Could you check a few things on this model? Use its own coordinates, in mm. Face numbers are marked on the shaded views. Coordinates: 2 decimals unless noted, no trailing zeros. Loops run counter-clockwise (first coordinate to the right, second up) from the corner with the lowest first, then second, coordinate; pieces in that order, holes last. Notation, with made-up numbers: (19.5, -4) -> (38.5, -4) arc R23 cw to (38.5, 8) -> close; hole circle Ø3 at (-4.75, 3). An arc over 180 degrees is marked (long way). One line per question, with ' | ' between items.
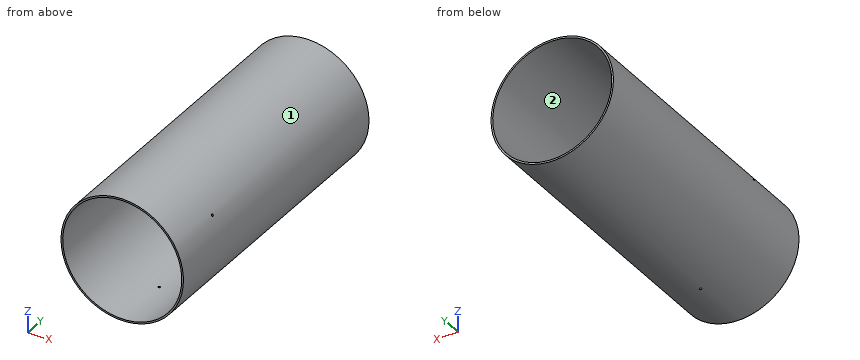
from build123d import *

# Parameters (mm, degrees)
SKETCH1_R               = 78.359
SKETCH1_R_2             = 76.2
BOSS_EXTRUDE1_DEPTH     = 381
CUT_EXTRUDE1_REACH      = 398.789
CUT_EXTRUDE1_END_RADIUS = 78.359
SKETCH2_R               = 1.41224
CIRPATTERN1_COUNT       = 3


with BuildPart() as part:
    # Sketch1 → Boss-Extrude1 (new body)
    with BuildSketch(Plane(origin=(0, 0, 0), x_dir=(1, 0, 0), z_dir=(0, 1, 0))):
        with Locations(Location((0, 0, 0), (0, 0, 270))):
            Circle(SKETCH1_R)
        with Locations(Location((0, 0, 0), (0, 0, 270))):
            Circle(SKETCH1_R_2, mode=Mode.SUBTRACT)
    extrude(amount=BOSS_EXTRUDE1_DEPTH)

    # Cut-Extrude1: up to this cylinder (the profile starts inside it)
    cut_extrude1_end = Plane(origin=(0, 76.2, 0), z_dir=(0, -1, 0)) * Cylinder(CUT_EXTRUDE1_END_RADIUS, 955.296, mode=Mode.PRIVATE)
    # Sketch2 → Cut-Extrude1 (cut, up to the surface)
    with BuildSketch(Plane.XY, mode=Mode.PRIVATE) as cut_extrude1_sk1:
        with Locations((0, 76.2)):
            Circle(SKETCH2_R)
    cut_extrude1_tool1 = extrude(cut_extrude1_sk1.sketch, amount=-CUT_EXTRUDE1_REACH, mode=Mode.PRIVATE) & cut_extrude1_end
    cut_extrude1 = cut_extrude1_tool1.solids().sort_by_distance((0, 76.2, 0))[0]
    add(cut_extrude1, mode=Mode.SUBTRACT)

    # CirPattern1: Cut-Extrude1 ×3 about axis
    cirpattern1_axis = Axis((0, 0, 0), (0, 1, 0))
    for i in range(1, CIRPATTERN1_COUNT):
        add(cut_extrude1.rotate(cirpattern1_axis, i * 360 / CIRPATTERN1_COUNT), mode=Mode.SUBTRACT)


solid = part.part
1) If we section it at A-A on x = 59.5: Please give me the cut outline in (y, z).
Data:
outline: (0, -50.99) -> (381, -50.99) -> (381, -47.6) -> (0, -47.6) -> close; (0, 47.6) -> (381, 47.6) -> (381, 50.99) -> (0, 50.99) -> close
2) If we section it at C-C on y = 303: Please give me the cut outline in (x, z), and give its area (3 significant figures).
Data:
outline: circle Ø156.72 at (0, 0); hole circle Ø152.4 at (0, 0) | area: 1,050 mm²
3) I'm going to push flat-ended pins straight in: pin 1 Ø1.5 at (x, y) = (54, 280) entering from -Z; pin 2 Ø3 at (y, z) = (166.5, 12) entering from -X; pin 3 Ø4 at (x, y) = (17.5, 103) entering from +Z; pin 4 Ø4 at (x, y) = (-2, 55) entering from -Z. Where does each tip first touch, or does it pass through?
Data:
pin 1: z = -57.49 | pin 2: x = -77.65 | pin 3: z = 76.81 | pin 4: z = -78.36
4) I need wall thicknesses on line 1 along Z through (x, y) = (0, 247); line 2 along X through (y, z) = (228.5, 3.5). Which ranges of each line are inside material? Lowest first, please. Write a range as from..to.
Data:
line 1: -78.36..-76.2, 76.2..78.36 | line 2: -78.28..-76.12, 76.12..78.28
5) If we section it at B-B on z = 0: Please give me the cut outline in (x, y).
Data:
outline: (-78.36, 0) -> (-76.2, 0) -> (-76.2, 381) -> (-78.36, 381) -> close; (76.2, 0) -> (78.36, 0) -> (78.36, 381) -> (76.2, 381) -> close
6) We'd pull the mould along X, two halves only. Please class the marked faces 1 and 2: pulls with the +X half, pulls with the -X half, needs draft (parallel to the pull), parting line crosses it, or undercut.
Data:
face 1: parting line crosses it | face 2: undercut
